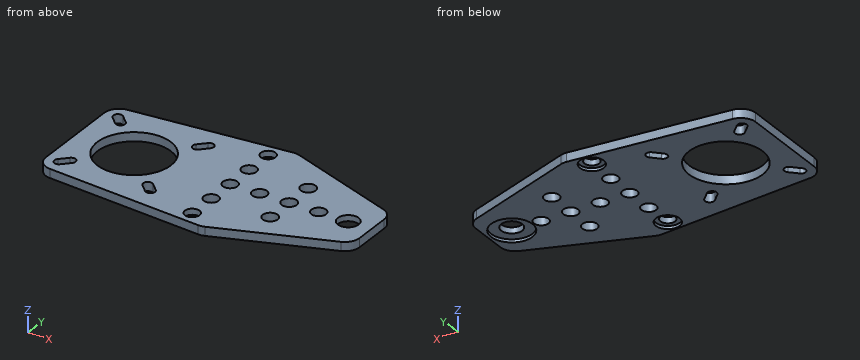
Autodesk Inventor part; units mm, degrees
ref_plane "YZ Plane" through (0, 0, 0) normal (1, 0, 0) x (0, 1, 0)
ref_plane "XZ Plane" through (0, 0, 0) normal (0, 1, 0) x (-1, 0, 0)
ref_plane "XY Plane" through (0, 0, 0) normal (0, 0, 1) x (1, 0, 0)
sketch "Sketch1" plane through (0, 0, 0) normal (0, 0, 1) x (1, 0, 0)
  circle A0 centre (80.14, 40.64) radius 3.57
  circle A1 centre (40.14, 40.64) radius 2.5
  circle A2 centre (40.14, 50.64) radius 2.5
  circle A3 centre (40.14, 60.64) radius 2.5
  circle A4 centre (40.14, 30.64) radius 2.5
  circle A5 centre (40.14, 20.64) radius 2.5
  circle A6 centre (7.59, 40.64) radius 12.5
  arc A7 (-4.314, 26.544) -> (-6.506, 28.736) centre (-5.41, 27.64) ccw
  line L0 (-6.814, 24.044) -> (-4.314, 26.544)
  arc A8 (-9.006, 26.236) -> (-6.814, 24.044) centre (-7.91, 25.14) ccw
  line L1 (-6.506, 28.736) -> (-9.006, 26.236)
  line L2 (-4.314, 54.736) -> (-6.814, 57.236)
  arc A9 (-6.506, 52.544) -> (-4.314, 54.736) centre (-5.41, 53.64) ccw
  line L3 (-9.006, 55.044) -> (-6.506, 52.544)
  arc A10 (-6.814, 57.236) -> (-9.006, 55.044) centre (-7.91, 56.14) ccw
  line L4 (21.994, 57.236) -> (19.494, 54.736)
  arc A11 (19.494, 54.736) -> (21.686, 52.544) centre (20.59, 53.64) ccw
  line L5 (21.686, 52.544) -> (24.186, 55.044)
  arc A12 (24.186, 55.044) -> (21.994, 57.236) centre (23.09, 56.14) ccw
  line L6 (24.186, 26.236) -> (21.686, 28.736)
  arc A13 (21.686, 28.736) -> (19.494, 26.544) centre (20.59, 27.64) ccw
  line L7 (19.494, 26.544) -> (21.994, 24.044)
  arc A14 (21.994, 24.044) -> (24.186, 26.236) centre (23.09, 25.14) ccw
  circle A15 centre (60.14, 40.64) radius 2.55
  circle A16 centre (60.14, 30.64) radius 2.55
  circle A17 centre (70.14, 40.64) radius 2.5
  circle A18 centre (60.14, 50.64) radius 2.55
  circle A19 centre (50.14, 40.64) radius 2.5
  line L8 (-12.41, 60.64) -> (-12.41, 20.64)
  line L9 (-12.41, 20.64) -> (46.5039, 15.4857)
  line L10 (46.5039, 15.4857) -> (88.14, 30.64)
  line L11 (88.14, 30.64) -> (88.14, 50.64)
  line L12 (88.14, 50.64) -> (46.5039, 65.7943)
  line L13 (46.5039, 65.7943) -> (-12.41, 60.64)
  point P0 (0, 0)
  dimension "d0" = 40
  dimension "d1" = 20
  dimension "d2" = 20
  dimension "d3" = 8
  dimension "d4" = 10
  dimension "d5" = 20
  dimension "d6" = 95
  dimension "d7" = 95
  dimension "d8" = 110
  dimension "d9" = 110
extrude "Extrusion1" add sketch "Sketch1" along normal blind 3
fillet "Fillet1" radius 5 6 edges at (-12.41, 20.64, 1.5) (46.5039, 15.4857, 1.5) (-12.41, 60.64, 1.5) (46.5039, 65.7943, 1.5) (88.14, 50.64, 1.5) (88.14, 30.64, 1.5)
sketch "Sketch2" plane through (0, 0, 0) normal (0, 0, -1) x (-1, 0, 0)
  circle A0 centre (-40.14, 20.64) radius 2.5
  circle A1 centre (-80.14, 40.64) radius 3.57
  circle A2 centre (-40.14, 60.64) radius 2.5
  point P0 (0, 0)
hole "Hole1" at (40.14, 20.64, 0) at (40.14, 60.64, 0) direction (0, 0, 1) diameter 8.1 depth 1
sketch "Sketch3" plane through (0, 0, 0) normal (0, 0, -1) x (-1, 0, 0)
  circle A0 centre (-80.14, 40.64) radius 3.57
  point P0 (0, 0)
hole "Hole2" at (80.14, 40.64, 0) direction (0, 0, 1) diameter 14 depth 1
equation "\"d7\" = d6"
properties part number "2020 Slider Motorized" material "Aluminum 6061"
Could you check a few things on this model? Use its own coordinates, in mm. Round coordinates to 2 decimals unless told otherwise and drop trailing zeros. Loops run counter-clockwise (first coordinate to the right, second up) from the corner with the lowest first, then second, coordinate; pieces in that order, holes last.
Q1. I want a section at A-A (y = 40.64). Give the number of separate pieces and of enclosed holes in the cut face, and give its area (3 significant figures).
Q2. I want a section at D-D (x = 5). Write out the boundary of the cut face in (y, z), and give its area (3 significant figures).
Q3. I want a section at C-C (y = 50.64). Write out the boundary of the cut face in (x, z), and give its area (3 significant figures).
Q4. I want a section at B-B (x = 60.14). Write out the boundary of the cut face in (y, z), and give its area (3 significant figures).
Q5. Please list where these lines run through material, in increasing order: L1, parallel to Y at x = 40.14, z = 0.7; L2, parallel to Y at x = 59, z = 2.3; L3, parallel to X at y = 32, z = 2.35.
Q6. For P1, Ø2.5, axis at x = 42, y = 22, coming from the -Z side; P2, Ø1.5, axis at x = 42.5, z = 2, coming from the +Y side; P3, Ø3, axis at x = 50.14, y = 40.64, coming from the +Z side, each with a flat end and sliding along its axis, tell me the tip position at first contact or that it passes through.
Answer below:
1. separate pieces: 7
1. enclosed holes: 0
1. area: 138 mm2
2. outline: (19.12, 0) - (28.41, 0) - (28.41, 3) - (19.12, 3) - close; (52.87, 0) - (62.16, 0) - (62.16, 3) - (52.87, 3) - close
2. area: 55.8 mm2
3. outline: (-12.41, 0) - (0.09, 0) - (0.09, 3) - (-12.41, 3) - close; (15.09, 0) - (37.64, 0) - (37.64, 3) - (15.09, 3) - close; (42.64, 0) - (57.59, 0) - (57.59, 3) - (42.64, 3) - close; (62.69, 0) - (86.71, 0) - (86.71, 3) - (62.69, 3) - close
3. area: 222 mm2
4. outline: (20.45, 0) - (28.09, 0) - (28.09, 3) - (20.45, 3) - close; (33.19, 0) - (38.09, 0) - (38.09, 3) - (33.19, 3) - close; (43.19, 0) - (48.09, 0) - (48.09, 3) - (43.19, 3) - close; (53.19, 0) - (60.83, 0) - (60.83, 3) - (53.19, 3) - close
4. area: 75.2 mm2
5. L1: y = 16.04 to 16.59, 24.69 to 28.14, 33.14 to 38.14, 43.14 to 48.14, 53.14 to 56.59, 64.69 to 65.24
5. L2: y = 20.03 to 28.36, 32.92 to 38.36, 42.92 to 48.36, 52.92 to 61.25
5. L3: x = -12.41 to -1.44, 16.62 to 38.04, 42.24 to 57.98, 62.3 to 87.66
6. P1: stops at z = 1
6. P2: stops at y = 65.51
6. P3: passes through
